Answer from the drawing. Dimensions are ordinates in mm from the lowest x, y and z of the part. A direction names the side the tool comes from. Give positions to 0.01 mm unless a question says otherwise; leave off trailing zeros. Loops run counter-clockwise (first coordinate to the right, second up) from the corner with the lowest first, then second, coordinate; pieces in that order, holes last. Notation, with made-up numbers: (24.5, 1.5) -> (75.5, 1.5) arc R20 cw to (75.5, 15.5) -> close; hole circle Ø3 at (54, 73.5). An arc over 180 degrees is marked (long way). Write each question's results on one line, items separated by ' | '. Start each with the question number.
Item 1: Determine the mould class of the marked faces 1 and 2 for opening direction X: +X half, -X half, draft (parallel to the pull), parting line (faces both ways), or undercut.
Item 2: Section C-C on z = 6.25 is taken. Write down the section's boundary in (x, y).
Item 3: Section A-A on x = 3.5 is taken. Write down the section's boundary in (y, z), and give its area (3 significant figures).
Item 4: Each of these flat-tipped pins is pushed along its axis until it touches: P1, Ø4, axis at x = 6.5, y = 3.5, coming from the -Z side; P2, Ø3, axis at y = 6, z = 5.5, coming from the +X side. Where does it stop, or does it pass through?
Item 5: Section D-D on y = 5.75 is taken. Write down the section's boundary in (x, z).
Item 6: Find the intervals of material crossed by line 1 (Y direction, x = 3.5, z = 4.85); line 2 (Z direction, x = 6.5, y = 4); line 3 (Z direction, x = 2.5, y = 5.25), in increasing order.
Item 7: Which of the six approach directions +Z, -Z, +X, -X, +Y, -Y give full straight-line access (tool end or side, diameter ignored) to the marked faces 3, 4 and 5?
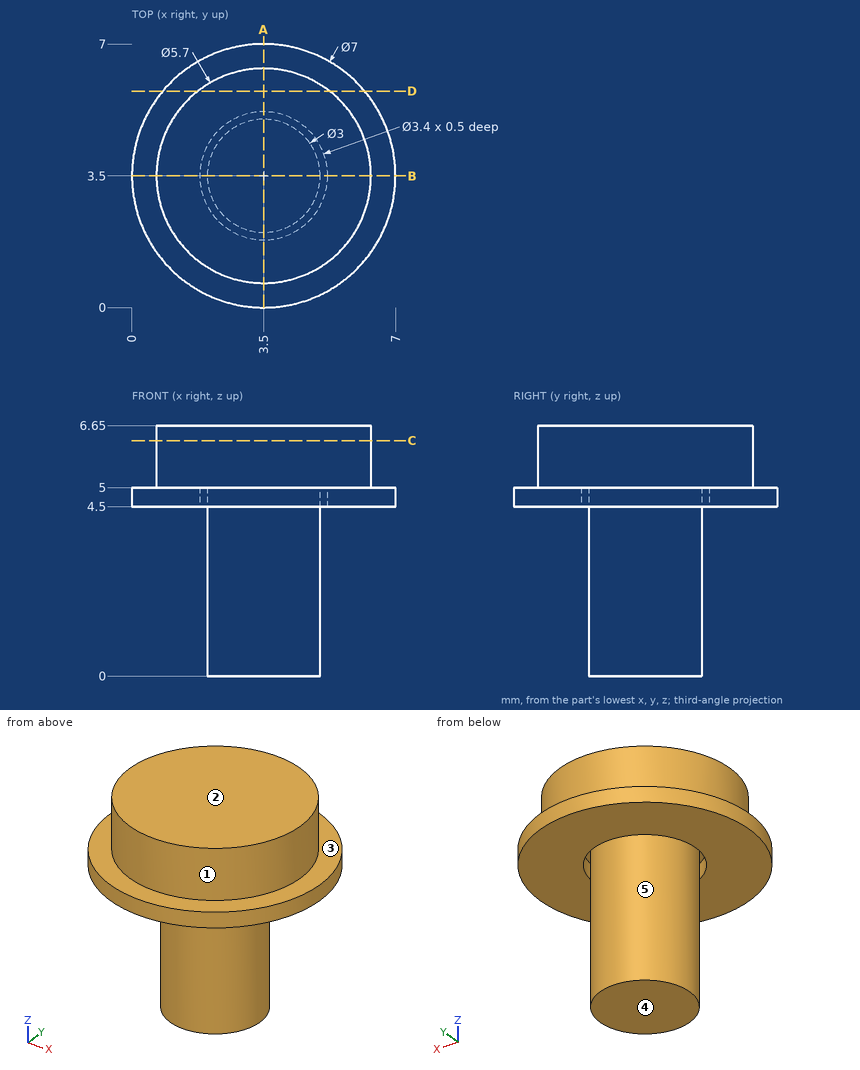
Findings:
1) face 1: parting line | face 2: draft
2) outline: circle Ø5.7 at (3.5, 3.5)
3) outline: (0, 4.5) -> (1.8, 4.5) -> (1.8, 5) -> (2, 5) -> (2, 0) -> (5, 0) -> (5, 5) -> (5.2, 5) -> (5.2, 4.5) -> (7, 4.5) -> (7, 5) -> (6.35, 5) -> (6.35, 6.65) -> (0.65, 6.65) -> (0.65, 5) -> (0, 5) -> close | area: 26.2 mm2
4) P1: z = 0 | P2: x = 6.83
5) outline: (0.82, 4.5) -> (6.18, 4.5) -> (6.18, 5) -> (5.25, 5) -> (5.25, 6.65) -> (1.75, 6.65) -> (1.75, 5) -> (0.82, 5) -> close
6) line 1: 0 to 1.8, 2 to 5, 5.2 to 7 | line 2: 4.5 to 5 | line 3: 4.5 to 6.65
7) face 3: +Z | face 4: -Z, +X, -X, +Y, -Y | face 5: -Z
